from build123d import *

# Parameters (mm, degrees)
SKETCH1_R               = 2
BOSS_EXTRUDE1_DEPTH     = 16
CUT_EXTRUDE1_DEPTH      = 17.248076809
CUT_EXTRUDE1_DEPTH_BACK = 17.248076809
SKETCH2_R               = 1
CHAMFER1_SIZE           = 0.5


with BuildPart() as part:
    # Sketch1 → Boss-Extrude1 (new body)
    with BuildSketch(Plane(origin=(0, 0, 0), x_dir=(0, 0, -1), z_dir=(1, 0, 0))):
        Circle(SKETCH1_R)
    extrude(amount=-BOSS_EXTRUDE1_DEPTH)

    # Sketch2 → Cut-Extrude1 (cut, two sides: drawn at the far end of the back side and taken through both)
    with BuildSketch(Plane(origin=(0, 0, 0), x_dir=(1, 0, 0), z_dir=(0, 1, 0)).offset(-CUT_EXTRUDE1_DEPTH_BACK)):
        with Locations(Location((-13.5, 0, 0), (0, 0, 270))):
            Circle(SKETCH2_R)
    extrude(amount=CUT_EXTRUDE1_DEPTH + CUT_EXTRUDE1_DEPTH_BACK, mode=Mode.SUBTRACT)

    # Sketch3 → Revolve1 (revolve)
    with BuildSketch(Plane(origin=(0, 0, 0), x_dir=(1, 0, 0), z_dir=(0, 1, 0))):
        with BuildLine():
            Line((0, 0), (0, -3.5))
            ThreePointArc((0, -3.5), (2.510871365, -2.481181976), (3.6, 0))
            Line((3.6, 0), (0, 0))
        make_face()
    revolve(axis=Axis((-3.287029336, 0, 0), (1, 0, 0)))

    # Chamfer1
    chamfer1_edges = [part.edges().sort_by_distance(p)[0] for p in [
        (-16, 0, 2),
    ]]
    chamfer(chamfer1_edges, length=CHAMFER1_SIZE)


solid = part.part
Geometry check sheet. Reference: the model listing, model coordinates, mm. Round coordinates to 2 decimals unless told otherwise and drop trailing zeros. Order: outer loops, then holes, each group sorted by start corner. A loop starts at its lowest first (then second) coordinate and runs counter-clockwise, first axis right, second up. Notation, with made-up numbers: (-30.75, -21.5) - (8.25, -21.5) arc R12 ccw to (8.25, -15.5) - close; hole circle Ø11 at (-8.5, -21). An arc over 180 degrees is marked (long way). One line per question, with ' | ' between items. Start each with the question number.
(1) Thickness scan on L1, parallel to X at y = -0.75, z = 0; L2, parallel to Z at x = -13.5, y = 0.35; L3, parallel to Z at x = -13.5, y = -0.7. Record the ranges inside material, lowest first. Write a range as [from, to].
(2) Depth check by flat-ended pin: pin 1 Ø1 at (y, z) = (-2.5, -1.5) entering from +X; pin 2 Ø1.2 at (x, z) = (-13.5, 0) entering from +Y; pin 3 Ø1.5 at (x, y) = (-2.5, 1.5) entering from +Z; pin 4 Ø1 at (y, z) = (-1, 0) entering from +X. Enter the tip coordinate at first touch or a pass-through.
(3) Sectioned sample at B-B on x = -13.75. Record the cut outline in (y, z), and give its area (3 significant figures).
(4) Sectioned sample at A-A on x = -9.75. Record the cut outline in (y, z).
(5) Release check for a two-part mould opening along X. For faces 1 (the flat face through (-16, 0, 0)), 2 (the cylindrical face through (-13.883, -0.028, 0.924)) record: released by +X, released by -X, zero draft, split by the parting line, or undercut.
Conclusion:
1) L1: x = [-16, -14.5], [-12.5, 3.5] | L2: z = [-1.97, -1], [1, 1.97] | L3: z = [-1.87, -1], [1, 1.87]
2) pin 1: stops at x = 2.58 | pin 2: passes through | pin 3: stops at z = 1.85 | pin 4: stops at x = 3.55
3) outline: (-1.75, -0.97) arc R2 ccw to (1.75, -0.97) - close; (-1.75, 0.97) - (1.75, 0.97) arc R2 ccw to start | area: 5.13 mm2
4) outline: circle Ø4 at (0, 0)
5) face 1: released by -X | face 2: undercut
